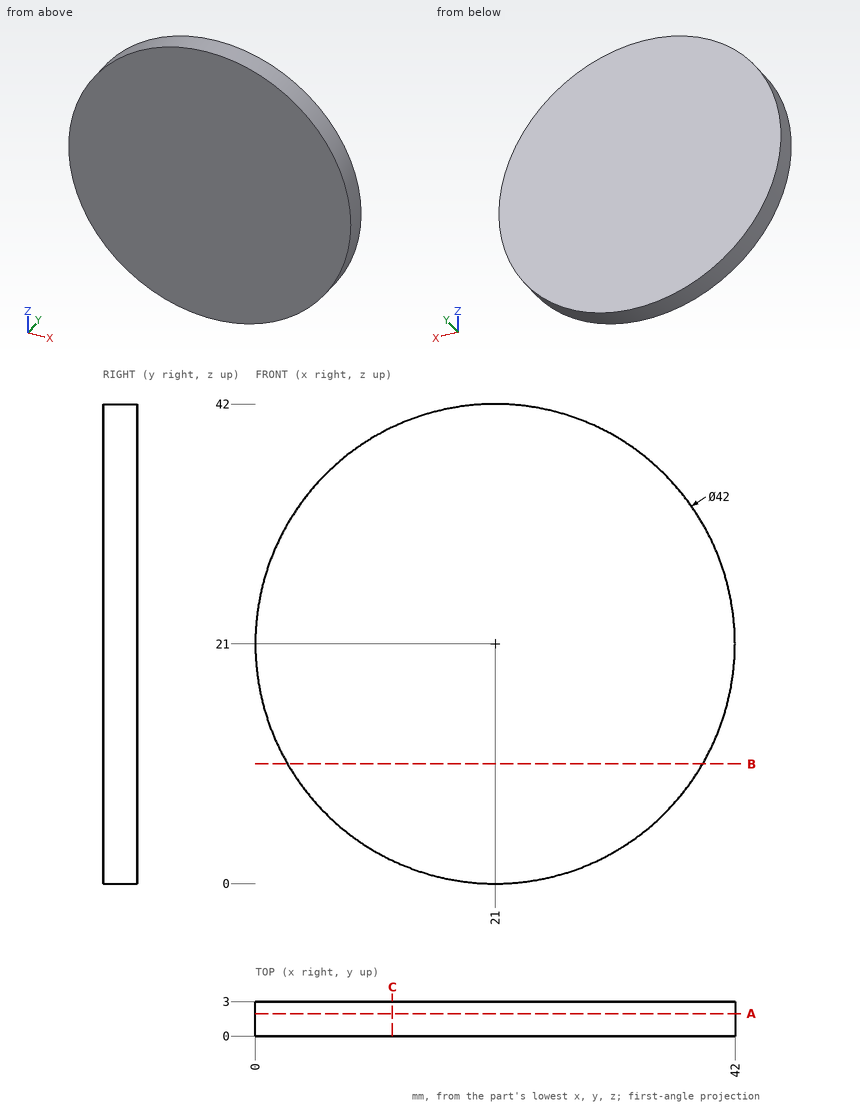
Input: dimensioned drawing with shaded views. Units: mm. Origin: part minimum x, y, z. Give positions to 0.01 mm unless a question says otherwise; leave off trailing zeros. Write each loop counter-clockwise with the first axis right and the second up, starting at its lowest first coordinate (ties: lowest second). Pieces come first, ordered by that corner, then holes. Notation, with made-up numbers: (9, -17) - (63, -17) arc R10 ccw to (63, 0) - close; hole circle Ø7 at (-12, -39). An arc over 180 degrees is marked (long way). One line per item, written item: value. Start each with the question number.
Q1. Material intervals for probe 1 along X at (y, z) = (0.85, 28); probe 2 along X at (y, z) = (0.9, 32), sorted ascending. Write a range as from..to.
Q2. Section query A-A, the plane y = 1.95. Return the cut outline in (x, z), then the cut area to 3 significant figures.
Q3. Section query C-C, the plane x = 12. Return the cut outline in (y, z).
Q4. First-contact query: pin 1 Ø1 at (x, y) = (6.5, 2.5) entering from -Z; pin 2 Ø1.5 at (y, z) = (1, 18.5) entering from -X. Flat tips, straight axial feed; report the tip coordinate or a pass-through.
Q5. Section query B-B, the plane z = 10.5. Return the cut outline in (x, y).
Answer:
1. probe 1: x = 1.2..40.8
1. probe 2: x = 3.11..38.89
2. outline: circle Ø42 at (21, 21)
2. area: 1,390 mm2
3. outline: (0, 2.03) - (3, 2.03) - (3, 39.97) - (0, 39.97) - close
4. pin 1: stops at z = 5.35
4. pin 2: stops at x = 0.07
5. outline: (2.81, 0) - (39.19, 0) - (39.19, 3) - (2.81, 3) - close
